The model under review builds one solid part; all positions refer to its coordinate system, in mm. Coordinates: 2 decimals unless noted, no trailing zeros. Loops run counter-clockwise (first coordinate to the right, second up) from the corner with the lowest first, then second, coordinate; pieces in that order, holes last. Notation, with made-up numbers: M -30,60.25 L 27,60.25 A19 cw 27,79.25 Z; hole C 11,-5 d6. An arc over 180 degrees is marked long. Return JSON: item names as keys, results as strings.
```python
from build123d import *

# Parameters (mm, degrees)
F0_W     = 100
F0_H     = 40
F1_DEPTH = 2
F2_W     = 79
F2_H     = 32
F2_W_2   = 71
F2_H_2   = 24
F3_DEPTH = 3.5
F4_W     = 65
F4_H     = 15
F5_DEPTH = 2
F6_SIZE  = 1.99999


# Not quite as in the source:
# - a fillet or chamfer is up to 0.001 mm smaller than in the source, because OpenCascade refuses the exact size


with BuildPart() as f1:
    # F0 (on Top) → F1 (new body)
    with BuildSketch(Plane.XY):
        Rectangle(F0_W, F0_H)
    extrude(amount=F1_DEPTH)

    # F2 (on face) → F3 (join)
    with BuildSketch(Plane.XY.offset(2)):
        Rectangle(F2_W, F2_H)
        Rectangle(F2_W_2, F2_H_2, mode=Mode.SUBTRACT)
    extrude(amount=F3_DEPTH)

    # F4 (on face) → F5 (cut, through all)
    with BuildSketch(Plane.XY.offset(2)):
        Rectangle(F4_W, F4_H)
    extrude(amount=-F5_DEPTH, mode=Mode.SUBTRACT)

    # F6 (size 2 in the source; OpenCascade refuses exactly that, so slightly less here)
    f6_edges = [f1.edges().sort_by_distance(p)[0] for p in [
        (32.5, 0, 0),
        (0, 7.5, 0),
        (-32.5, 0, 0),
        (0, -7.5, 0),
        (0, 20, 0),
        (50, 0, 0),
        (0, -20, 0),
        (-50, 0, 0),
    ]]
    chamfer(f6_edges, length=F6_SIZE)


solid = f1.part
```
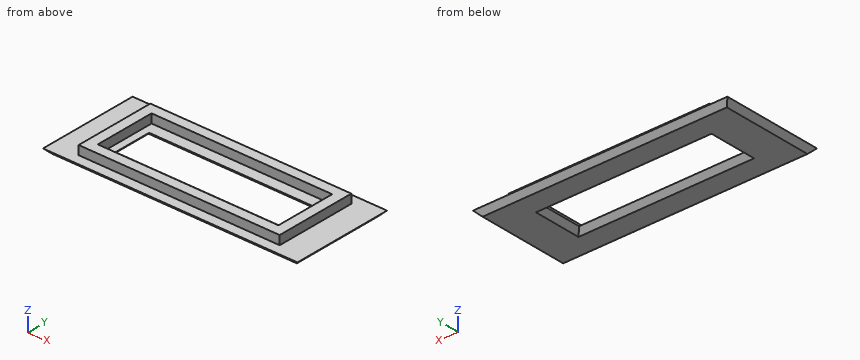
1. Insertion check: pin 1 Ø3 at (x, z) = (-6, 4.5) entering from -Y; pin 2 Ø1 at (y, z) = (-3.5, 4) entering from +X; pin 3 Ø1.8 at (y, z) = (-4.5, 4.5) entering from -X; pin 4 Ø12 at (x, y) = (5.5, -0.5) entering from +Z. Each pin has a flat end and moves straight along its axis. Give the tip position at first contact, or say it passes through.
Check values:
{"pin 1": "y = -16", "pin 2": "x = 39.5", "pin 3": "x = -39.5", "pin 4": "through"}
2. Add section A-A on z = 3. Give the boundary of the cut face in (x, y).
Check values:
{"outline": "M -39.5,-16 L 39.5,-16 L 39.5,16 L -39.5,16 Z; hole M -35.5,-12 L 35.5,-12 L 35.5,12 L -35.5,12 Z"}
3. To check wall thickness, follow line 1 (Y direction, x = 11, z = 4.65); line 2 (X direction, y = 7, z = 3.1); line 3 (Y direction, x = -37, z = 4.15). State the ranges of each line that lie inside material, in increasing order.
Check values:
{"line 1": "-16 to -12, 12 to 16", "line 2": "-39.5 to -35.5, 35.5 to 39.5", "line 3": "-16 to 16"}
